The model under review builds one solid part; all positions refer to its coordinate system, in mm. Face numbers are marked on the shaded views. A direction names the side the tool comes from. Coordinates: 2 decimals unless noted, no trailing zeros. Loops run counter-clockwise (first coordinate to the right, second up) from the corner with the lowest first, then second, coordinate; pieces in that order, holes last. Notation, with made-up numbers: (-32.5, 43.25) - (14.5, 43.25) arc R26 cw to (14.5, 59.25) - close; hole circle Ø7 at (9, 71). An arc over 180 degrees is marked (long way). Use a Markdown table: item, result. Add a question column.
1) Clearance check with flat-ended pins moving along their axes: pin 1 (24 mm diameter, centred on x = 70.5, z = 52, fed in from -Y); pin 2 (4 mm diameter, centred on x = 49.5, y = 38.5, fed in from -Z); pin 3 (8 mm diameter, centred on y = 25, z = 45.5, fed in from +X); pin 4 (10 mm diameter, centred on y = 24.5, z = 59.5, fed in from +X). State where each tip first meets the part, or that it passes through.
2) Add section A-A, the plane z = 74. Give the boundary of the cut face in (x, y), and give its area (3 significant figures).
3) To check wall thickness, follow L1, parallel to Z at x = 72, y = 25; L2, parallel to Z at x = 31, y = 41; L3, parallel to Y at x = 68.5, z = 13.5. State the ranges of each line that lie inside material, in increasing order. Write a range as [from, to].
4) Add section D-D, the plane y = 4.5. Give the boundary of the cut face in (x, z).
5) Add section B-B, the plane z = 55. Give the boundary of the cut face in (x, y), and give its area (3 significant figures).
6) The part is to be moulded in two halves that separate along X. For the marked faces 1, 2 and 3, say which applies: pulls with the +X half, pulls with the -X half, needs draft (parallel to the pull), parting line crosses it, or undercut.
7) For the marked faces 4, 5, 6 and 7, list the 3-axis set-ups (+Z, -Z, +X, -X, +Y, -Y) from which the entire face can be reached by the end or side of a thin tool; tool diameter is ignored.
8) Add section C-C, the plane x = 67. Give the boundary of the cut face in (y, z), and give its area (3 significant figures).
```python
from build123d import *

# Parameters (mm, degrees)
F0_W      = 100
F0_H      = 45
F1_DEPTH  = 100
F3_DEPTH  = 40
F4_W      = 45
F4_H      = 20
F5_DEPTH  = 100.001
F7_DEPTH  = 100.001
F9_DEPTH  = 85
F10_W     = 30
F10_H     = 30
F11_DEPTH = 10


with BuildPart() as f1:
    # F0 (on Top) → F1 (new body)
    with BuildSketch(Plane.XY):
        with Locations((50, 22.5)):
            Rectangle(F0_W, F0_H)
    extrude(amount=F1_DEPTH)

    # F2 (on face) → F3 (cut)
    with BuildSketch(Plane.XY.offset(100)):
        Polygon((35, 45), (15, 45), (0, 20), (0, 0), (35, 0), align=None)
    extrude(amount=-F3_DEPTH, mode=Mode.SUBTRACT)

    # F4 (on face) → F5 (cut, through all)
    with BuildSketch(Plane.XY.offset(100)):
        with Locations((57.5, 10)):
            Rectangle(F4_W, F4_H)
    extrude(amount=-F5_DEPTH, mode=Mode.SUBTRACT)

    # F6 (on face) → F7 (cut, through all)
    with BuildSketch(Plane.XY.offset(100)):
        Polygon((100, 45), (80, 20), (80, 0), (100, 0), align=None)
    extrude(amount=-F7_DEPTH, mode=Mode.SUBTRACT)

    # F8 (on face) → F9 (cut)
    with BuildSketch(Plane.XY.offset(100)):
        Polygon((50, 45), (35, 45), (35, 21), align=None)
    extrude(amount=-F9_DEPTH, mode=Mode.SUBTRACT)

    # F10 (on face) → F11 (cut)
    with BuildSketch(Plane.XZ.offset(-20)):
        with Locations((70, 45)):
            Rectangle(F10_W, F10_H)
    extrude(amount=-F11_DEPTH, mode=Mode.SUBTRACT)


solid = f1.part
```
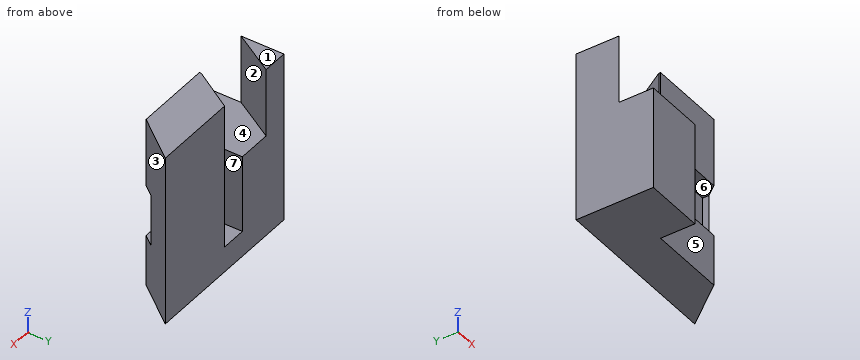
From the geometry:
| question | item | result |
|---|---|---|
| 1 | pin 1 | stops at y = 20 |
| 1 | pin 2 | stops at z = 0 |
| 1 | pin 3 | stops at x = 87.2 |
| 1 | pin 4 | stops at x = 87.6 |
| 2 | outline | (0, 20) - (15, 45) - (0, 45) - close; (35, 20) - (80, 20) - (100, 45) - (50, 45) - (35, 21) - close |
| 2 | area | 1,380 mm^2 |
| 3 | L1 | z = [0, 30], [60, 100] |
| 3 | L2 | z = [0, 60] |
| 3 | L3 | y = [20, 45] |
| 4 | outline | (0, 0) - (35, 0) - (35, 60) - (0, 60) - close |
| 5 | outline | (0, 0) - (35, 0) - (35, 20) - (55, 20) - (55, 30) - (85, 30) - (85, 26.25) - (100, 45) - (50, 45) - (35, 21) - (35, 45) - (0, 45) - close |
| 5 | area | 2,490 mm^2 |
| 6 | face 1 | needs draft |
| 6 | face 2 | undercut |
| 6 | face 3 | pulls with the +X half |
| 7 | face 4 | +Z, -Y |
| 7 | face 5 | +Z, -Z, +X, -Y |
| 7 | face 6 | -Y |
| 7 | face 7 | +Z, +Y |
| 8 | outline | (20, 0) - (45, 0) - (45, 100) - (20, 100) - (20, 60) - (30, 60) - (30, 30) - (20, 30) - close |
| 8 | area | 2,200 mm^2 |
